Autodesk Inventor part; units mm, degrees
ref_plane "YZ Plane" through (0, 0, 0) normal (1, 0, 0) x (0, 1, 0)
ref_plane "XZ Plane" through (0, 0, 0) normal (0, 1, 0) x (-1, 0, 0)
ref_plane "XY Plane" through (0, 0, 0) normal (0, 0, 1) x (1, 0, 0)
sketch "Sketch1" plane through (0, 0, 0) normal (0, 1, 0) x (-1, 0, 0)
  line L0 (0, 820) -> (0, 0)
  line L1 (760, 796.5895) -> (760, 820)
  line L2 (760, 820) -> (0, 820)
  line L3 (760, 796.5895) -> (110, 0)
  line L4 (110, 0) -> (0, 0)
  line L5 (758.3, 820) -> (755.9389, 786.2346)
  line L6 (755.9389, 786.2346) -> (686.7934, 701.4952)
  line L7 (686.7934, 701.4952) -> (684.7101, 704.3201)
  line L8 (663.2335, 678) -> (0, 678)
  dimension "d1" = 760
  dimension "d2" = 23.411
  dimension "d5" = 129.214
  dimension "d6" = 110
  dimension "d7" = 1.7
  dimension "d8" = 3.4
  dimension "d9" = 820
  dimension "d10" = 4
  dimension "d11" = 109.37
  dimension "d12" = 75.621
  dimension "d22" = 678
extrude "Plate1" add sketch "Sketch1" along normal blind 2 contours L8 L3 L4 L0
mirror "Mirror1" about plane through (0, 0, 0) normal (1, 0, 0)
sketch "Sketch2" plane through (0, 0, 0) normal (0, -1, 0) x (1, 0, 0)
  line L0 (-110, 0) -> (110, 0) construction
  line L1 (-110, 0) -> (-663.2335, 678) construction
  circle A0 centre (-305.821, 432.1909) radius 84.5
  line L2 (-663.2335, 678) -> (663.2335, 678)
  line L3 (110, 0) -> (663.2335, 678) construction
  circle A1 centre (0, 150) radius 84.5
  circle A2 centre (315.3114, 606.7132) radius 44.75
  line L4 (-110, 0) -> (110, 0) construction
  line L5 (-221.321, 432.1909) -> (-221.321, 136.4263) construction
  line L6 (-84.5, 150) -> (-84.5, -31.2508) construction
  line L7 (84.5, 150) -> (84.5, 0) construction
  line L8 (270.5614, 606.7132) -> (270.5614, 0) construction
  line L9 (-305.821, 516.6909) -> (270.5614, 516.6909) construction
  line L10 (-305.821, 347.6909) -> (270.5614, 347.6909) construction
  line L11 (0, 234.5) -> (270.5614, 234.5) construction
  line L12 (315.3114, 561.9632) -> (270.5614, 561.9632) construction
  point P0 (0, 0)
  point P1 (0, 0)
  point P2 (0, 0)
  point P3 (0, 0)
  point P4 (-84.5, 59.3746)
  dimension "d13" = 169
  dimension "d16" = 150
  dimension "d17" = 432.191
  dimension "d18" = 305.821
  dimension "d19" = 113.191
  dimension "d20" = 89.5
  dimension "d21" = 136.821
extrude "Extrusion1" cut sketch "Sketch2" against normal through all
equation "\"d3\" = Thickness"
equation "\"BendRadius\" = Thickness"
equation "\"BendReliefWidth\" = Thickness"
equation "\"BendReliefDepth\" = 0.5 * Thickness"
equation "\"CornerReliefSize\" = 4 * Thickness"
equation "\"MinimumRemnant\" = 2 * Thickness"
equation "\"TransitionRadius\" = BendRadius"
equation "\"JacobiRadiusSize\" = BendRadius"
equation "\"GapSize\" = Thickness"
properties part number "МОО 073 face 3"
Verification items for the finished model (mm, model axes). Give positions to 0.01 mm unless a question says otherwise; leave off trailing zeros. Write each loop counter-clockwise with the first axis right and the second up, starting at its lowest first coordinate (ties: lowest second). Pieces come first, ordered by that corner, then holes. Notation, with made-up numbers: M -4,29.25 L 20,29.25 A30 cw 20,61.25 Z; hole C 74.25,65.5 d4. An arc over 180 degrees is marked long. Write item = value, one per line.
(1) Material ranges on line 1 (Z direction, x = 0, y = 1.65); line 2 (X direction, y = 1.6, z = 154); line 3 (X direction, y = 1.4, z = 502.5), recorded low to high.
Found:
line_1 = 0 to 65.5, 234.5 to 678
line_2 = -235.66 to -84.41, 84.41 to 235.66
line_3 = -520.03 to -352.69, -258.95 to 520.03
(2) Sectioned sample at B-B (z = 150). Record the cut outline in (x, y), then the cut area to 3 significant figures.
Found:
outline = M -232.4,0 L -84.5,0 L -84.5,2 L -232.4,2 Z; M 84.5,0 L 232.4,0 L 232.4,2 L 84.5,2 Z
area = 592 mm2
(3) Sectioned sample at D-D (x = 150). Record the cut outline in (y, z), then the cut area to 3 significant figures.
Found:
outline = M 0,49.02 L 2,49.02 L 2,678 L 0,678 Z
area = 1,260 mm2
(4) Draft check along Z on faces 1 (the face through (-260.39, 0.99, 503.44)), 2 (the face through (9, 0, 419)), 3 (the face through (-390.489, 0.986, 343.746)). Enter one of: released by +Z, released by -Z, zero draft, split by the parting line, or undercut.
Found:
face_1 = undercut
face_2 = zero draft
face_3 = released by -Z
(5) Sectioned sample at C-C (y = 0.55). Record the cut outline in (x, z), then the cut area to 3 significant figures.
Found:
outline = M -663.23,678 L -110,0 L 110,0 L 663.23,678 Z; hole C -305.82,432.19 d169; hole C 0,150 d169; hole C 315.31,606.71 d89.5
area = 473,000 mm2
(6) Sectioned sample at A-A (x = 0). Record the cut outline in (y, z).
Found:
outline = M 0,0 L 2,0 L 2,65.5 L 0,65.5 Z; M 0,234.5 L 2,234.5 L 2,678 L 0,678 Z
